Here's how the part is built. I have some questions about the finished solid (model axes, mm). A direction names the side the tool comes from. Coordinates: 2 decimals unless noted, no trailing zeros. Write each loop counter-clockwise with the first axis right and the second up, starting at its lowest first coordinate (ties: lowest second). Pieces come first, ordered by that corner, then holes. Notation, with made-up numbers: (14, 8) -> (52, 8) arc R9 cw to (52, 22) -> close; hole circle Ø4 at (5, 56.25). An arc over 180 degrees is marked (long way). Use a Markdown table: item, result. Add a question column.
Item 1: On a 3-axis mill with a long thin cutter (end or side, diameter ignored), from which of +Z, -Z, +X, -X, +Y, -Y can I reach the whole of each face in a straight line? I mean faces 5 (the flat face through (10.576, 1.498, 0.74)), 6 (the flat face through (13.262, 17, 2)), 7 (the flat face through (7.562, 17, 2)). Say none if no direction works.
Item 2: Imagine slicing it at A-A, the plane x = 11.5. Write out the boundary of the cut face in (y, z), and give its area (3 significant figures).
Item 3: If we mould it in two halves opening along X, with no side actions, what happens to faces 1 (the flat face through (7.576, 1.498, 0.74)), 2 (the flat face through (18.312, 13, 1)), 3 (the flat face through (3.234, 1.541, 0.74)), 4 (the flat face through (9, 10, 0))? For each: pulls with the +X half, pulls with the -X half, needs draft (parallel to the pull), parting line crosses it, or undercut.
Item 4: If I drill on line 1 along X through (y, z) = (1.75, 0.95); line 2 along Z through (x, y) = (3, 8.75); line 3 along Y through (x, z) = (8.25, 2.1), over which ranges is the centre line in solid material (lowest first)? Write a range as from..to.
Item 5: Imagine slicing it at C-C, the plane z = 1.9. Write out the boundary of the cut face in (x, y), and give its area (3 significant figures).
Item 6: Will these pins go through, and if not, where does the flat tip stop? pin 1 Ø0.6 at (x, z) = (8.5, 1) entering from -Y; pin 2 Ø0.8 at (x, z) = (11.5, 0.5) entering from -Y; pin 3 Ø1 at (y, z) = (13.5, 1.5) entering from -X.
Item 7: Imagine slicing it at D-D, the plane x = 3.75. Write out the boundary of the cut face in (y, z), and give its area (4 significant figures).
Item 8: Imagine slicing it at B-B, the plane y = 16.75. Write out the boundary of the cut face in (x, z).
```python
from build123d import *

# Parameters (mm, degrees)
BOSS_EXTRUDE1_DEPTH = 1.5
RGB_LED_W           = 5.7
RGB_LED_H           = 3.7
BOSS_EXTRUDE2_DEPTH = 1


with BuildPart() as part:
    # Sketch1 → Boss-Extrude1 (new body)
    with BuildSketch(Plane.XY):
        Polygon((0, 6), (0.314446676, 0), (1.497941481, 0), (1.657221927, 3.039251967), (2.042586863, 3.65596478), (2.769801294, 3.65596478), (3.155166229, 3.039251967), (3.314446676, 0), (4.497941481, 0), (4.657221927, 3.039251967), (5.042586863, 3.65596478), (5.769801294, 3.65596478), (6.155166229, 3.039251967), (6.314446676, 0), (7.497941481, 0), (7.657221927, 3.039251967), (8.042586863, 3.65596478), (8.769801294, 3.65596478), (9.155166229, 3.039251967), (9.314446676, 0), (10.497941481, 0), (10.657221927, 3.039251967), (11.042586863, 3.65596478), (11.769801294, 3.65596478), (12.155166229, 3.039251967), (12.314446676, 0), (13.497941481, 0), (13.657221927, 3.039251967), (14.042586863, 3.65596478), (16.269801294, 3.65596478), (16.655166229, 3.039251967), (16.814446676, 0), (17.997941481, 0), (18.312388157, 6), (18.312388157, 19.7), (0, 19.7), align=None)
    extrude(amount=BOSS_EXTRUDE1_DEPTH)

    # rgb_led → Boss-Extrude2 (add)
    with BuildSketch(Plane.XY.offset(1.5)):
        with Locations((10.412388157, 16.9)):
            Rectangle(RGB_LED_W, RGB_LED_H)
    extrude(amount=BOSS_EXTRUDE2_DEPTH)


solid = part.part
```
Ans:
| question | item | result |
|---|---|---|
| 1 | face 5 | +Z, -Z, -Y |
| 1 | face 6 | +Z, +X, +Y, -Y |
| 1 | face 7 | +Z, -X, +Y, -Y |
| 2 | outline | (3.66, 0) -> (19.7, 0) -> (19.7, 1.5) -> (18.75, 1.5) -> (18.75, 2.5) -> (15.05, 2.5) -> (15.05, 1.5) -> (3.66, 1.5) -> close |
| 2 | area | 27.8 mm^2 |
| 3 | face 1 | undercut |
| 3 | face 2 | pulls with the +X half |
| 3 | face 3 | undercut |
| 3 | face 4 | needs draft |
| 4 | line 1 | x = 0.22..1.59, 3.22..4.59, 6.22..7.59, 9.22..10.59, 12.22..13.59, 16.72..18.09 |
| 4 | line 2 | z = 0..1.5 |
| 4 | line 3 | y = 15.05..18.75 |
| 5 | outline | (7.56, 15.05) -> (13.26, 15.05) -> (13.26, 18.75) -> (7.56, 18.75) -> close |
| 5 | area | 21.1 mm^2 |
| 6 | pin 1 | stops at y = 3.61 |
| 6 | pin 2 | stops at y = 3.45 |
| 6 | pin 3 | stops at x = 0 |
| 7 | outline | (0, 0) -> (19.7, 0) -> (19.7, 1.5) -> (0, 1.5) -> close |
| 7 | area | 29.55 mm^2 |
| 8 | outline | (0, 0) -> (18.31, 0) -> (18.31, 1.5) -> (13.26, 1.5) -> (13.26, 2.5) -> (7.56, 2.5) -> (7.56, 1.5) -> (0, 1.5) -> close |
